Check sheet for the modelled part. Datum: model origin and axes. Units: mm. A direction names the side the tool comes from. Give positions to 0.01 mm unless a question says otherwise; leave off trailing zeros. Loops run counter-clockwise (first coordinate to the right, second up) from the corner with the lowest first, then second, coordinate; pieces in that order, holes last. Notation, with made-up numbers: (58.25, -33) -> (104.25, -33) arc R26 cw to (104.25, -7) -> close; hole circle Ø7 at (-36.75, 45). An arc over 180 degrees is marked (long way). Write each question's results on one line, items separated by ' | '. Start each with the question number.
Item 1: Access from +Z, -Z, +X, -X, +Y, -Y to the whole of each face (thin tool, end or side, straight path). Record for faces 1 (the face through (17.71, 2.31, 14.95)), 2 (the face through (-25.27, 19.26, -2.38)), 3 (the face through (1, 1, 17.1)).
Item 2: Cross-section at C-C on z = 21. Enter the section's corners in (x, y), then the cut area to 3 significant figures.
Item 3: Scan lines: line 1 along Z through (x, y) = (-13.5, 5); line 2 along Y through (x, z) = (-24.75, 15.5); line 3 along Y through (x, z) = (-25.3, -15.5). Record each from-to range of solid material in increasing order.
Item 4: Gauge pin test, flat ends, axial feed: pin 1 Ø3 at (y, z) = (7.5, -18.5) entering from +X; pin 2 Ø6 at (x, z) = (10, -12.5) entering from +Y. Record the tip position at first contact, or that the pin passes through.
Item 5: Mould release check, pull along Z, two halves, no side actions. Record for faces 4 (the face through (-25, 49, -22)), 5 (the face through (-23.4, 3.07, 0.35)), 6 (the face through (17.6, 1.3, 15)), 7 (the face through (0, 1, 12.9)): pulls with the +Z half, pulls with the -Z half, needs draft (parallel to the pull), parting line crosses it, or undercut.
Item 6: Cross-section at B-B on y = 14.5. Enter the section's corners in (x, z).
Item 7: Cross-section at A-A on x = 3. Enter the section's corners in (y, z), then the cut area to 3 significant figures.
Item 8: Cross-section at D-D on y = 8.5. Enter the section's corners in (x, z).
from build123d import *

# Parameters (mm, degrees)
SKETCH1_W           = 53
SKETCH1_H           = 50
BOSS_EXTRUDE1_DEPTH = 2.5
SKETCH2_W           = 50
SKETCH2_H           = 51
BOSS_EXTRUDE2_DEPTH = 2.5
CHAMFER1_SIZE       = 5
SKETCH3_R           = 11
SKETCH3_R_2         = 2
CUT_EXTRUDE1_DEPTH  = 2.5
CUT_EXTRUDE2_DEPTH  = 2.5
FILLET1_R           = 2
FILLET2_R           = 2
CHAMFER2_SIZE       = 0.3
CHAMFER3_SIZE       = 0.3
BOSS_EXTRUDE3_DEPTH = 2.5
BOSS_EXTRUDE4_DEPTH = 2.5


with BuildPart() as part:
    # Sketch1 → Boss-Extrude1 (new body)
    with BuildSketch(Plane(origin=(0, 0, 0), x_dir=(1, 0, 0), z_dir=(0, 1, 0))):
        Rectangle(SKETCH1_W, SKETCH1_H)
    extrude(amount=BOSS_EXTRUDE1_DEPTH)

    # Sketch2 → Boss-Extrude2 (add)
    with BuildSketch(Plane.ZY.offset(26.5)):
        with Locations((0, 25.5)):
            Rectangle(SKETCH2_W, SKETCH2_H)
    extrude(amount=-BOSS_EXTRUDE2_DEPTH)

    # Chamfer1
    chamfer1_edges = [part.edges().sort_by_distance(p)[0] for p in [
        (-25.25, 51, 25),
        (-25.25, 51, -25),
        (26.5, 1.25, 25),
        (26.5, 1.25, -25),
    ]]
    chamfer(chamfer1_edges, length=CHAMFER1_SIZE)

    # Sketch3 → Cut-Extrude1 (cut)
    with BuildSketch(Plane.ZY.offset(26.5)):
        with Locations((0, 30)):
            Circle(SKETCH3_R)
        with Locations((-15.5, 45.5)):
            Circle(SKETCH3_R_2)
        with Locations((15.5, 45.5)):
            Circle(SKETCH3_R_2)
        with Locations((-15.5, 14.5)):
            Circle(SKETCH3_R_2)
        with Locations((15.5, 14.5)):
            Circle(SKETCH3_R_2)
    extrude(amount=-CUT_EXTRUDE1_DEPTH, mode=Mode.SUBTRACT)

    # Sketch4 → Cut-Extrude2 (cut)
    with BuildSketch(Plane(origin=(0, 2.5, 0), x_dir=(1, 0, 0), z_dir=(0, 1, 0))):
        with BuildLine():
            Line((-14.5, 17.1), (15.5, 17.1))
            ThreePointArc((15.5, 17.1), (17.6, 15), (15.5, 12.9))
            Line((15.5, 12.9), (-14.5, 12.9))
            ThreePointArc((-14.5, 12.9), (-16.6, 15), (-14.5, 17.1))
        make_face()
        with BuildLine():
            Line((-14.5, -12.9), (15.5, -12.9))
            ThreePointArc((15.5, -12.9), (17.6, -15), (15.5, -17.1))
            Line((15.5, -17.1), (-14.5, -17.1))
            ThreePointArc((-14.5, -17.1), (-16.6, -15), (-14.5, -12.9))
        make_face()
    extrude(amount=-CUT_EXTRUDE2_DEPTH, mode=Mode.SUBTRACT)

    # Fillet1
    fillet1_edges = [part.edges().sort_by_distance(p)[0] for p in [
        (-24, 2.5, 0),
    ]]
    fillet(fillet1_edges, radius=FILLET1_R)

    # Fillet2
    fillet2_edges = [part.edges().sort_by_distance(p)[0] for p in [
        (-26.5, 0, 0),
    ]]
    fillet(fillet2_edges, radius=FILLET2_R)

    # Chamfer2
    chamfer2_edges = [part.edges().sort_by_distance(p)[0] for p in [
        (-24, 45.5, -17.5),
        (-26.5, 45.5, -17.5),
        (-24, 45.5, 13.5),
        (-26.5, 45.5, 13.5),
        (-24, 14.5, -17.5),
        (-26.5, 14.5, -17.5),
        (-24, 14.5, 13.5),
        (-26.5, 14.5, 13.5),
    ]]
    chamfer(chamfer2_edges, length=CHAMFER2_SIZE)

    # Chamfer3
    chamfer3_edges = [part.edges().sort_by_distance(p)[0] for p in [
        (-16.6, 0, 15),
        (0.5, 2.5, 12.9),
        (17.6, 0, 15),
        (0.5, 0, 17.1),
        (0.5, 0, 12.9),
        (-16.6, 2.5, 15),
        (0.5, 2.5, 17.1),
        (17.6, 2.5, 15),
        (-16.6, 0, -15),
        (0.5, 2.5, -17.1),
        (17.6, 0, -15),
        (0.5, 0, -12.9),
        (0.5, 0, -17.1),
        (-16.6, 2.5, -15),
        (0.5, 2.5, -12.9),
        (17.6, 2.5, -15),
    ]]
    chamfer(chamfer3_edges, length=CHAMFER3_SIZE)

    # Sketch5 → Boss-Extrude3 (add)
    with BuildSketch(Plane.XY.offset(25)):
        Polygon((-24, 22.5), (-11, 2.5), (-21.171930363, 2.5), (-24, 6.850876365), align=None)
    extrude(amount=-BOSS_EXTRUDE3_DEPTH)

    # Sketch6 → Boss-Extrude4 (add)
    with BuildSketch(Plane(origin=(0, 0, -25), x_dir=(-1, 0, 0), z_dir=(0, 0, -1))):
        Polygon((24, 22.5), (11, 2.5), (21.171930363, 2.5), (24, 6.850876365), align=None)
    extrude(amount=-BOSS_EXTRUDE4_DEPTH)


solid = part.part
Answer sheet:
1) face 1: +Y | face 2: +X, -X | face 3: +Y, -Y
2) outline: (-26.5, 2) arc R2 ccw to (-24.5, 0) -> (25.5, 0) -> (25.5, 2.5) -> (-22, 2.5) arc R2 cw to (-24, 4.5) -> (-24, 50) -> (-26.5, 50) -> close | area: 249 mm²
3) line 1: z = -25 to -22.5, 22.5 to 25 | line 2: y = 0.02 to 12.5, 16.5 to 43.5, 47.5 to 51 | line 3: y = 0.17 to 12.5, 16.5 to 43.5, 47.5 to 51
4) pin 1: stops at x = -24 | pin 2: stops at y = 2.5
5) face 4: pulls with the -Z half | face 5: needs draft | face 6: undercut | face 7: undercut
6) outline: (-26.5, -25) -> (-18.8, -25) -> (-18.8, -22.5) -> (-24, -22.5) -> (-24, -17.8) -> (-24.3, -17.5) -> (-26.2, -17.5) -> (-26.5, -17.8) -> close; (-26.5, -13.2) -> (-26.2, -13.5) -> (-24.3, -13.5) -> (-24, -13.2) -> (-24, 13.2) -> (-24.3, 13.5) -> (-26.2, 13.5) -> (-26.5, 13.2) -> close; (-26.5, 17.8) -> (-26.2, 17.5) -> (-24.3, 17.5) -> (-24, 17.8) -> (-24, 22.5) -> (-18.8, 22.5) -> (-18.8, 25) -> (-26.5, 25) -> close
7) outline: (0, -25) -> (2.5, -25) -> (2.5, -17.4) -> (2.2, -17.1) -> (0.3, -17.1) -> (0, -17.4) -> close; (0, -12.6) -> (0.3, -12.9) -> (2.2, -12.9) -> (2.5, -12.6) -> (2.5, 12.6) -> (2.2, 12.9) -> (0.3, 12.9) -> (0, 12.6) -> close; (0, 17.4) -> (0.3, 17.1) -> (2.2, 17.1) -> (2.5, 17.4) -> (2.5, 25) -> (0, 25) -> close | area: 104 mm²
8) outline: (-26.5, -25) -> (-14.9, -25) -> (-14.9, -22.5) -> (-24, -22.5) -> (-24, 22.5) -> (-14.9, 22.5) -> (-14.9, 25) -> (-26.5, 25) -> close
